from build123d import *

# Parameters (mm, degrees)
F0_R     = 3
F1_DEPTH = 19.65
F2_R     = 7


with BuildPart() as f1:
    # F0 (on Front) → F1 (new body)
    with BuildSketch(Plane.XZ):
        with BuildLine():
            ThreePointArc((0, 17.5), (17.5, 0), (0, -17.5))
            Line((0, -17.5), (-250, -17.5))
            Line((-250, -17.5), (-250, -32.5))
            Line((-250, -32.5), (0, -32.5))
            ThreePointArc((0, -32.5), (32.5, 0), (0, 32.5))
            Line((0, 32.5), (-70, 32.5))
            Line((-70, 32.5), (-70, 17.5))
            Line((-70, 17.5), (0, 17.5))
        make_face()
        with Locations((-242, -25)):
            Circle(F0_R, mode=Mode.SUBTRACT)
        with Locations((-62, 25)):
            Circle(F0_R, mode=Mode.SUBTRACT)
    extrude(amount=F1_DEPTH)

    # F2
    f2_edges = [f1.edges().sort_by_distance(p)[0] for p in [
        (-250, -9.825, -17.5),
        (-250, -9.825, -32.5),
        (-70, -9.825, 17.5),
        (-70, -9.825, 32.5),
    ]]
    fillet(f2_edges, radius=F2_R)


solid = f1.part
The model under review builds one solid part; all positions refer to its coordinate system, in mm. A direction names the side the tool comes from. Coordinates: 2 decimals unless noted, no trailing zeros. Loops run counter-clockwise (first coordinate to the right, second up) from the corner with the lowest first, then second, coordinate; pieces in that order, holes last.
(1) Draft analysis for pull direction Z (two halves, no side actions). For faces 1 (the cylindrical face through (17.496, -9.687, 0.385)), 2 (the flat face through (-78, -19.65, -19)), 3 (the cylindrical face through (-68, -10, 30.4)), state which applies: +Z half, -Z half, draft (parallel to the pull), parting line (faces both ways), or undercut.
Determined:
face 1: undercut
face 2: draft
face 3: +Z half
(2) Insertion check: P1, Ø1.5, axis at y = -12.5, z = -7.5, coming from the +X side; P2, Ø1.1, axis at y = -5.5, z = 25, coming from the -X side; P3, Ø8, axis at y = -16.5, z = 20.5, coming from the +X side. Each pin has a flat end and moves straight along its axis. Give the tip position at first contact, or say it passes through.
Determined:
P1: stops at x = 31.79
P2: stops at x = -70
P3: stops at x = 28
(3) Consider section A-A, the plane y = -16.25. Give the boundary of the cut face in (x, z), plus the area to 3 significant figures.
Determined:
outline: (-250, -25.5) arc R7 ccw to (-243, -32.5) - (0, -32.5) arc R32.5 ccw to (0, 32.5) - (-63, 32.5) arc R7 ccw to (-70, 25.5) - (-70, 24.5) arc R7 ccw to (-63, 17.5) - (0, 17.5) arc R17.5 cw to (0, -17.5) - (-243, -17.5) arc R7 ccw to (-250, -24.5) - close; hole circle Ø6 at (-242, -25); hole circle Ø6 at (-62, 25)
area: 5,880 mm2
(4) Tool access review of faces 4 (the cylindrical face through (-247.9, -10, -19.5)), 5 (the cylindrical face through (-67.9, -10, 19.5)): name each direction out of +Z, -Z, +X, -X, +Y, -Y from which nothing blocks a thin tool from reaching the whole face with its end or side.
Determined:
face 4: +Z, -X, +Y, -Y
face 5: -X, +Y, -Y
(5) Wall thickness on L1, parallel to Z at x = -62, y = -11.75; L2, parallel to Z at x = -40, y = -12; L3, parallel to Z at x = -242, y = -4.75: over which ranges is each line inside the solid? List them lowest first.
Determined:
L1: z = -32.5 to -17.5, 17.5 to 22, 28 to 32.5
L2: z = -32.5 to -17.5, 17.5 to 32.5
L3: z = -32.5 to -28, -22 to -17.5
(6) Consider section B-B, the plane x = -120. Give the boundary of the cut face in (y, z).
Determined:
outline: (-19.65, -32.5) - (0, -32.5) - (0, -17.5) - (-19.65, -17.5) - close
(7) Consider section C-C, the plane z = 0. Give the boundary of the cut face in (x, y).
Determined:
outline: (17.5, -19.65) - (32.5, -19.65) - (32.5, 0) - (17.5, 0) - close
